from build123d import *

# Parameters (mm, degrees)
SKETCH1_R               = 4
BOSS_EXTRUDE1_DEPTH     = 2
CUT_EXTRUDE1_DEPTH      = 121.138144992
CUT_EXTRUDE1_DEPTH_BACK = 121.138144992
SKETCH2_R               = 6


with BuildPart() as part:
    # Sketch1 → Boss-Extrude1 (new body)
    with BuildSketch(Plane.XY):
        with BuildLine():
            Line((-16.429017806, -29.488280523), (-10, 108.982872222))
            ThreePointArc((-10, 108.982872222), (0, 118.982872222), (10, 108.982872222))
            Line((10, 108.982872222), (16.429017806, -29.488280523))
            ThreePointArc((16.429017806, -29.488280523), (0, -47.517127778), (-16.429017806, -29.488280523))
        make_face()
        with Locations((0, 40.242872222)):
            Circle(SKETCH1_R, mode=Mode.SUBTRACT)
    extrude(amount=BOSS_EXTRUDE1_DEPTH)

    # Sketch2 → Cut-Extrude1 (cut, two sides: drawn at the far end of the back side and taken through both)
    with BuildSketch(Plane.XY.offset(2).offset(-CUT_EXTRUDE1_DEPTH_BACK)):
        with Locations((0, -31.017127778)):
            Circle(SKETCH2_R)
    extrude(amount=CUT_EXTRUDE1_DEPTH + CUT_EXTRUDE1_DEPTH_BACK, mode=Mode.SUBTRACT)


solid = part.part
The listing builds one solid part. Answer for the finished solid, in the listing's coordinates (mm). Round coordinates to 2 decimals unless told otherwise and drop trailing zeros. Order: outer loops, then holes, each group sorted by start corner. A loop starts at its lowest first (then second) coordinate and runs counter-clockwise, first axis right, second up. Notation, with made-up numbers: (-27.75, 22.5) -> (-3.75, 22.5) arc R29 cw to (-3.75, 58.5) -> close; hole circle Ø8 at (34.5, -2). An arc over 180 degrees is marked (long way). Write each question's results on one line, items separated by ' | '. Start each with the question number.
Q1. The mould has two halves that part along X. Classify faces 1 (the cylindrical face through (-1.301, -36.874, 0.986)), 2 (the flat face through (-13.26, 38.78, 0.99)), 3 (the cylindrical face through (-0.52, 44.21, 0.99)), 4 (the cylindrical face through (-0.22, 118.98, 0.99)): pulls with the +X half, pulls with the -X half, needs draft (parallel to the pull), parting line crosses it, or undercut.
Q2. Find section A-A (x = 0). Determine the outline of the cut face in (y, z).
Q3. Find section D-D (x = 14.5). Determine the outline of the cut face in (y, z), then the cut area to 3 significant figures.
Q4. Find section C-C (y = -12). Determine the outline of the cut face in (x, z).
Q5. Straight lines are drawn through the part: probe 1 along Y at (x, z) = (0, 0.8); probe 2 along Y at (x, z) = (-2.5, 1.2); probe 3 along X at (y, z) = (-31.5, 0.7). For each, find the intervals that lie inside material, in ascending order. Write a range as from..to.
Q6. Find section B-B (z = 1.35). Determine the outline of the cut face in (x, y), then the cut area to 3 significant figures.
Worked answers:
1) face 1: undercut | face 2: pulls with the -X half | face 3: undercut | face 4: parting line crosses it
2) outline: (-47.52, 0) -> (-37.02, 0) -> (-37.02, 2) -> (-47.52, 2) -> close; (-25.02, 0) -> (36.24, 0) -> (36.24, 2) -> (-25.02, 2) -> close; (44.24, 0) -> (118.98, 0) -> (118.98, 2) -> (44.24, 2) -> close
3) outline: (-38.89, 0) -> (12.06, 0) -> (12.06, 2) -> (-38.89, 2) -> close | area: 102 mm2
4) outline: (-15.62, 0) -> (15.62, 0) -> (15.62, 2) -> (-15.62, 2) -> close
5) probe 1: y = -47.52..-37.02, -25.02..36.24, 44.24..118.98 | probe 2: y = -47.33..-36.47, -25.56..37.12, 43.37..118.67 | probe 3: x = -16.49..-5.98, 5.98..16.49
6) outline: (-16.43, -29.49) arc R16.5 ccw (long way) to (16.43, -29.49) -> (10, 108.98) arc R10 ccw to (-10, 108.98) -> close; hole circle Ø12 at (0, -31.02); hole circle Ø8 at (0, 40.24) | area: 4,130 mm2
